from build123d import *

# Parameters (mm, degrees)
SKETCH_1_W          = 10
SKETCH_1_H          = 22
EXTRUDE_1_DEPTH     = 30
SKETCH_2_W          = 6
SKETCH_2_H          = 6
EXTRUDE_3_DEPTH     = 14
SKETCH_3_R          = 1.5
CUT_EXTRUDE_1_DEPTH = 6
SKETCH_6_W          = 10
SKETCH_6_H          = 30
CUT_EXTRUDE_2_DEPTH = 2
SKETCH_7_W          = 6
SKETCH_7_H          = 6
EXTRUDE_4_DEPTH     = 2
FILLET_1_R          = 1
SKETCH_8_R          = 1.6
CUT_EXTRUDE_3_DEPTH = 4


with BuildPart() as part:
    # 草图1 → 凸台-拉伸1 (new body)
    with BuildSketch(Plane.XY):
        with Locations((5, 11)):
            Rectangle(SKETCH_1_W, SKETCH_1_H)
    extrude(amount=EXTRUDE_1_DEPTH)

    # 草图2 → 凸台-拉伸3 (add)
    with BuildSketch(Plane.XY):
        with Locations((5, 12)):
            Rectangle(SKETCH_2_W, SKETCH_2_H)
    extrude(amount=-EXTRUDE_3_DEPTH)

    # 草图3 → 切除-拉伸1 (cut)
    with BuildSketch(Plane(origin=(0, 9, 0), x_dir=(-1, 0, 0), z_dir=(0, -1, 0))):
        with Locations(Location((-5, 11, 0), (0, 0, 90))):
            Circle(SKETCH_3_R)
    extrude(amount=-CUT_EXTRUDE_1_DEPTH, mode=Mode.SUBTRACT)

    # 草图6 → 切除-拉伸2 (cut)
    with BuildSketch(Plane(origin=(0, 22, 0), x_dir=(1, 0, 0), z_dir=(0, 1, 0))):
        with Locations((5, -15)):
            Rectangle(SKETCH_6_W, SKETCH_6_H)
    extrude(amount=-CUT_EXTRUDE_2_DEPTH, mode=Mode.SUBTRACT)

    # 草图7 → 凸台-拉伸4 (add)
    with BuildSketch(Plane(origin=(0, 0, -14), x_dir=(-1, 0, 0), z_dir=(0, 0, -1))):
        with Locations((-5, 12)):
            Rectangle(SKETCH_7_W, SKETCH_7_H)
    extrude(amount=EXTRUDE_4_DEPTH)

    # 圆角1
    fillet_1_edges = [part.edges().sort_by_distance(p)[0] for p in [
        (10, 10, 30),
        (2, 9, -8),
        (2, 15, -8),
        (8, 15, -8),
        (8, 9, -8),
        (2, 12, 0),
        (5, 9, 0),
        (8, 12, 0),
        (5, 15, 0),
        (0, 10, 30),
        (0, 10, 0),
        (0, 20, 15),
        (5, 20, 0),
        (10, 20, 15),
        (5, 20, 30),
        (2, 12, -16),
        (5, 15, -16),
        (8, 12, -16),
        (5, 9, -16),
        (10, 10, 0),
        (5, 0, 0),
        (10, 0, 15),
        (0, 0, 15),
        (5, 0, 30),
    ]]
    fillet(fillet_1_edges, radius=FILLET_1_R - 0.0001)  # a hair under: the kernel refuses the full size

    # 草图8 → 切除-拉伸3 (cut)
    with BuildSketch(Plane(origin=(0, 0, -16), x_dir=(-1, 0, 0), z_dir=(0, 0, -1))):
        with Locations((-5, 12)):
            Circle(SKETCH_8_R)
    extrude(amount=-CUT_EXTRUDE_3_DEPTH, mode=Mode.SUBTRACT)


solid = part.part
Check sheet for the modelled part. Datum: model origin and axes. Units: mm. A direction names the side the tool comes from. Round coordinates to 2 decimals unless told otherwise and drop trailing zeros. Order: outer loops, then holes, each group sorted by start corner. A loop starts at its lowest first (then second) coordinate and runs counter-clockwise, first axis right, second up. Notation, with made-up numbers: M 30.25,31.25 L 87.25,31.25 A21 ccw 87.25,67.25 Z; hole C 32,25 d3. An arc over 180 degrees is marked long. One line per item, written item: value. Start each with the question number.
1. Section check D-D on z = -5. Enter the section's corners in (x, y).
2. Access from +Z, -Z, +X, -X, +Y, -Y to the whole of each face (thin tool, end or side, straight path). Record for faces 4 (the cylindrical face through (2.285, 12.028, -15.699)), 5 (the cylindrical face through (2.285, 14.699, -7.902)), 6 (the flat face through (8, 12, -8)), 7 (the cylindrical face through (7.715, 14.699, -7.902)), 8 (the flat face through (5, 15, -8)).
3. Section check A-A on x = 5. Enter the section's corners in (y, z).
4. Release check for a two-part mould opening along Y. For faces 1 (the cylindrical face through (5.208, 13.586, -14.028)), 2 (the flat face through (5, 20, 15)), 3 (the cylindrical face through (7.715, 12.028, -15.699)) record: released by +Y, released by -Y, zero draft, split by the parting line, or undercut.
5. Scan lines: line 1 along X through (y, z) = (13.5, -11); line 2 along Y through (x, z) = (5, -13.2); line 3 along X through (y, z) = (12, -14.25). Record each from-to range of solid material in increasing order.
6. Gauge pin test, flat ends, axial feed: P1, Ø2, axis at x = 3.5, z = -8.5, coming from the -Y side; P2, Ø4.5, axis at x = 5, z = -5, coming from the +Y side; P3, Ø1.2, axis at y = 12.5, z = -8.5, coming from the -X side. Record the tip position at first contact, or that the pin passes through.
7. Section check B-B on z = -11. Enter the section's corners in (x, y), and give its area (3 significant figures).
Results found:
1. outline: M 2,10 A1 ccw 3,9 L 7,9 A1 ccw 8,10 L 8,14 A1 ccw 7,15 L 3,15 A1 ccw 2,14 Z
2. face 4: -Z, -X, +Y, -Y
2. face 5: -Z, -X, +Y
2. face 6: -Z, +X, +Y, -Y
2. face 7: -Z, +X, +Y
2. face 8: -Z, +X, -X, +Y
3. outline: M 0,1 A1 ccw 1,0 L 8,0 A1 cw 9,-1 L 9,-9.5 L 15,-9.5 L 15,-1 A1 cw 16,0 L 19,0 A1 ccw 20,1 L 20,29 A1 ccw 19,30 L 1,30 A1 ccw 0,29 Z; M 9,-15 A1 ccw 10,-16 L 10.4,-16 L 10.4,-12.5 L 9,-12.5 Z; M 13.6,-16 L 14,-16 A1 ccw 15,-15 L 15,-12.5 L 13.6,-12.5 Z
4. face 1: undercut
4. face 2: released by +Y
4. face 3: zero draft
5. line 1: 2 to 3.5, 6.5 to 8
5. line 2: 9 to 10.4, 13.6 to 15
5. line 3: 2 to 3.4, 6.6 to 8
6. P1: y = 9
6. P2: y = 15
6. P3: x = 2
7. outline: M 2,10 A1 ccw 3,9 L 3.5,9 L 3.5,15 L 3,15 A1 ccw 2,14 Z; M 6.5,9 L 7,9 A1 ccw 8,10 L 8,14 A1 ccw 7,15 L 6.5,15 Z
7. area: 17.1 mm^2
